Build history of the part. All positions in model axes, mm. A direction names the side the tool comes from. Coordinates: 2 decimals unless noted, no trailing zeros. Loops run counter-clockwise (first coordinate to the right, second up) from the corner with the lowest first, then second, coordinate; pieces in that order, holes last.
(1) Slice it at D-D (z = 62). Give the cut face in (x, y), and give its area (3 significant figures).
(2) Slice it at A-A (z = 26.5). Give the cut face in (x, y), and give its area (3 significant figures).
(3) Slice it at B-B (x = 88.5). Give the cut face in (y, z), and give its area (3 significant figures).
(4) Slice it at C-C (y = 8.5). Give the number of separate pieces and of enclosed holes in the cut face, and give its area (3 significant figures).
(5) Tool access for faces 5 (the face through (-126, 5, 20)), 6 (the face through (36, 10, -2)), 7 (the face through (-20, 5, -126)): list every direction of +Z, -Z, +X, -X, +Y, -Y with a clear straight run to the whole face (end or side of a thin tool).
(6) Flat gauge pins, fed straight in: P1, Ø1, axis at x = -45.5, y = 1.5, coming from the -Z side; P2, Ø4, axis at x = -64.5, y = 3.5, coming from the +Z side; P3, Ø5, axis at x = 34, y = 1.5, coming from the +Z side. Where does each tip first touch, or does it go through?
(7) Wall check: L1, parallel to X at y = 3, z = 0; L2, parallel to X at y = 9.5, z = -16; L3, parallel to X at y = 1.5, z = 30.5. Give the ranges that are in metal, low to high.
(8) Two-plate mould, pull along X, no slides. Class faces 1 (the face through (36, 0, -2)), 2 (the face through (76.47, 5.07, -72.88)), 3 (the face through (141.96, 5.07, -0.81)), 4 (the face through (20, 5, -126)): pulls with the +X half, pulls with the -X half, needs draft (parallel to the pull), parting line crosses it, or undercut.
from build123d import *

# Parameters (mm, degrees)
SKETCH1_R           = 155
BOSS_EXTRUDE1_DEPTH = 10
SKETCH2_R           = 6.25
CUT_EXTRUDE1_DEPTH  = 220.431082575
SKETCH3_R           = 35
CUT_EXTRUDE2_DEPTH  = 220.431082575
SKETCH4_R           = 3.05
CUT_EXTRUDE3_DEPTH  = 220.431082575
CIRPATTERN1_COUNT   = 8
CUT_EXTRUDE4_START  = -10
CUT_EXTRUDE4_DEPTH  = 10
CIRPATTERN3_COUNT   = 4
FILLET1_R           = 20
CUT_EXTRUDE5_DEPTH  = 218.60055147


with BuildPart() as part:
    # Sketch1 → Boss-Extrude1 (new body)
    with BuildSketch(Plane(origin=(0, 0, 0), x_dir=(1, 0, 0), z_dir=(0, 1, 0))):
        with Locations(Location((0, 0, 0), (0, 0, 270))):
            Circle(SKETCH1_R)
    extrude(amount=BOSS_EXTRUDE1_DEPTH)

    # Sketch2 → Cut-Extrude1 (cut, through all)
    with BuildSketch(Plane(origin=(0, 10, 0), x_dir=(1, 0, 0), z_dir=(0, 1, 0))):
        with Locations(Location((-135.764501988, 0, 0), (0, 0, 270))):
            Circle(SKETCH2_R)
        with Locations(Location((0, -135.764501988, 0), (0, 0, 270))):
            Circle(SKETCH2_R)
        with Locations(Location((135.764501988, 0, 0), (0, 0, 270))):
            Circle(SKETCH2_R)
        with Locations(Location((0, 135.764501988, 0), (0, 0, 270))):
            Circle(SKETCH2_R)
    extrude(amount=-CUT_EXTRUDE1_DEPTH, mode=Mode.SUBTRACT)

    # Sketch3 → Cut-Extrude2 (cut, through all)
    with BuildSketch(Plane(origin=(0, 10, 0), x_dir=(1, 0, 0), z_dir=(0, 1, 0))):
        with Locations(Location((0, 0, 0), (0, 0, 270))):
            Circle(SKETCH3_R)
    extrude(amount=-CUT_EXTRUDE2_DEPTH, mode=Mode.SUBTRACT)

    # Sketch4 → Cut-Extrude3 (cut, through all)
    with BuildSketch(Plane(origin=(0, 10, 0), x_dir=(1, 0, 0), z_dir=(0, 1, 0))):
        with Locations(Location((17.220754456, 41.574578963, 0), (0, 0, 270))):
            Circle(SKETCH4_R)
    cut_extrude3 = extrude(amount=-CUT_EXTRUDE3_DEPTH, mode=Mode.SUBTRACT)

    # CirPattern1: Cut-Extrude3 ×8 about axis
    cirpattern1_axis = Axis((0, 0, 0), (0, 1, 0))
    for i in range(1, CIRPATTERN1_COUNT):
        add(cut_extrude3.rotate(cirpattern1_axis, i * 360 / CIRPATTERN1_COUNT), mode=Mode.SUBTRACT)

    # Sketch5 → Cut-Extrude4 (cut)
    with BuildSketch(Plane(origin=(0, 10, 0), x_dir=(1, 0, 0), z_dir=(0, 1, 0)).offset(CUT_EXTRUDE4_START)):
        with BuildLine():
            Line((-153.704261489, 20), (-118.321595662, 20))
            ThreePointArc((-118.321595662, 20), (-84.852813742, 84.852813742), (-20, 118.321595662))
            Line((-20, 118.321595662), (-20, 153.704261489))
            ThreePointArc((-20, 153.704261489), (-109.601551084, 109.601551084), (-153.704261489, 20))
        make_face()
        with BuildLine():
            Line((-153.704261489, -20), (-153.704261489, 20))
            ThreePointArc((-153.704261489, 20), (-155, 0), (-153.704261489, -20))
        make_face()
    cut_extrude4 = extrude(amount=CUT_EXTRUDE4_DEPTH, mode=Mode.SUBTRACT)

    # CirPattern3: Cut-Extrude4 ×4 about axis
    cirpattern3_axis = Axis((0, 0, 0), (0, 1, 0))
    for i in range(1, CIRPATTERN3_COUNT):
        add(cut_extrude4.rotate(cirpattern3_axis, i * 360 / CIRPATTERN3_COUNT), mode=Mode.SUBTRACT)

    # Fillet1
    fillet1_edges = [part.edges().sort_by_distance(p)[0] for p in [
        (-153.704261489, 5, -20),
        (-20, 5, 153.704261489),
        (153.704261489, 5, 20),
        (20, 5, -153.704261489),
        (-153.704261489, 5, 20),
        (20, 5, 153.704261489),
        (153.704261489, 5, -20),
        (-20, 5, -153.704261489),
    ]]
    fillet(fillet1_edges, radius=FILLET1_R - 0.0001)  # a hair under: the kernel refuses the full size

    # Sketch6 → Cut-Extrude5 (cut, through all)
    with BuildSketch(Plane(origin=(0, 10, 0), x_dir=(1, 0, 0), z_dir=(0, 1, 0))):
        Polygon((77.781745931, 77.781745931), (68.122487668, 75.193555479), (75.193555479, 68.122487668), align=None)
    extrude(amount=-CUT_EXTRUDE5_DEPTH, mode=Mode.SUBTRACT)


solid = part.part
Response values:
1. outline: (-102.74, 0) - (102.74, 0) - (102.74, 10) - (-102.74, 10) - close
1. area: 2,050 mm2
2. outline: (-117.04, 0) - (-22.86, 0) - (-22.86, 10) - (-117.04, 10) - close; (22.86, 0) - (117.04, 0) - (117.04, 10) - (22.86, 10) - close
2. area: 1,880 mm2
3. outline: (0, -81.04) - (10, -81.04) - (10, 81.04) - (0, 81.04) - close
3. area: 1,620 mm2
4. separate pieces: 1
4. enclosed holes: 14
4. area: 45,400 mm2
5. face 5: +Z, -X, +Y, -Y
5. face 6: +Z, -Z, +X, -X, +Y
5. face 7: -Z, -X, +Y, -Y
6. P1: stops at z = -111.24
6. P2: stops at z = 102.44
6. P3: stops at z = 115.79
7. L1: x = -153.7 to -142.01, -129.51 to -35, 35 to 129.51, 142.01 to 153.7
7. L2: x = -145.7 to -44.37, -38.78 to -31.13, 31.13 to 38.78, 44.37 to 145.7
7. L3: x = -116.06 to -17.17, 17.17 to 116.06
8. face 1: needs draft
8. face 2: undercut
8. face 3: undercut
8. face 4: pulls with the +X half
